```python
from build123d import *

# Parameters (mm, degrees)
SKETCH1_W                    = 400
SKETCH1_H                    = 150
BASE_FLANGE1_DEPTH           = 3
EDGE_FLANGE1_STRIP_W         = 13.4732
EDGE_FLANGE1_STRIP_H         = 3
EDGE_FLANGE1_STRIP_CUT_DEPTH = 400
EDGE_FLANGE1_DEPTH           = 400
EDGE_FLANGE2_STRIP_W         = 13.4732
EDGE_FLANGE2_STRIP_H         = 3
EDGE_FLANGE2_STRIP_CUT_DEPTH = 400
EDGE_FLANGE2_DEPTH           = 400


# Sheet-metal steps are written as plain solids
with BuildPart() as part:
    # Sketch1 → Base-Flange1 (new body)
    with BuildSketch(Plane.XY):
        Rectangle(SKETCH1_W, SKETCH1_H)
    extrude(amount=-BASE_FLANGE1_DEPTH)

    # Edge-Flange1 strip (across the edge) → Edge-Flange1 strip cut (cut)
    with BuildSketch(Plane(origin=(-200, -75, 0), x_dir=(0, 1, 0), z_dir=(1, 0, 0))):
        with Locations((-3, -1.5)):
            Rectangle(EDGE_FLANGE1_STRIP_W, EDGE_FLANGE1_STRIP_H)
    extrude(amount=EDGE_FLANGE1_STRIP_CUT_DEPTH, mode=Mode.SUBTRACT)

    # Edge-Flange1 section (across the edge) → Edge-Flange1 (add)
    with BuildSketch(Plane(origin=(-200, -75, 0), x_dir=(0, 1, 0), z_dir=(1, 0, 0))):
        with BuildLine():
            Line((0, 0.7366), (0, 50.8))
            Line((0, 50.8), (3, 50.8))
            Line((3, 50.8), (3, 0.7366))
            ThreePointArc((3, 0.7366), (3.215745145, 0.215745145), (3.7366, 0))
            Line((3.7366, 0), (3.7366, -3))
            ThreePointArc((3.7366, -3), (1.094424801, -1.905575199), (0, 0.7366))
        make_face()
    extrude(amount=EDGE_FLANGE1_DEPTH)

    # Edge-Flange2 strip (across the edge) → Edge-Flange2 strip cut (cut)
    with BuildSketch(Plane(origin=(200, 75, 0), x_dir=(0, -1, 0), z_dir=(-1, 0, 0))):
        with Locations((-3, -1.5)):
            Rectangle(EDGE_FLANGE2_STRIP_W, EDGE_FLANGE2_STRIP_H)
    extrude(amount=EDGE_FLANGE2_STRIP_CUT_DEPTH, mode=Mode.SUBTRACT)

    # Edge-Flange2 section (across the edge) → Edge-Flange2 (add)
    with BuildSketch(Plane(origin=(200, 75, 0), x_dir=(0, -1, 0), z_dir=(-1, 0, 0))):
        with BuildLine():
            Line((0, 0.7366), (0, 50.8))
            Line((0, 50.8), (3, 50.8))
            Line((3, 50.8), (3, 0.7366))
            ThreePointArc((3, 0.7366), (3.215745145, 0.215745145), (3.7366, 0))
            Line((3.7366, 0), (3.7366, -3))
            ThreePointArc((3.7366, -3), (1.094424801, -1.905575199), (0, 0.7366))
        make_face()
    extrude(amount=EDGE_FLANGE2_DEPTH)


solid = part.part
```
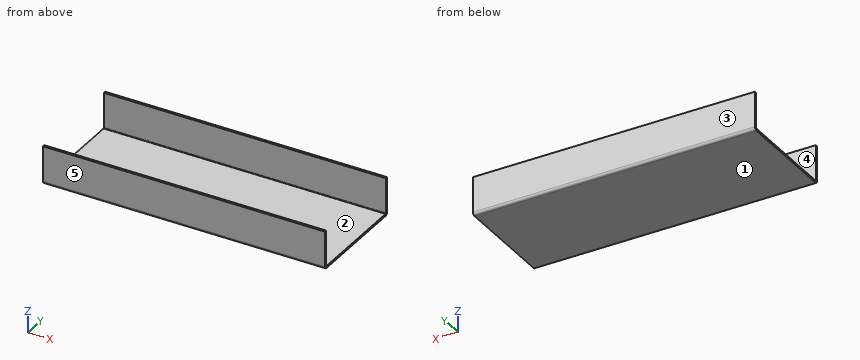
Check sheet for the modelled part. Datum: model origin and axes. Units: mm. Face numbers are marked on the shaded views. A direction names the side the tool comes from. Round coordinates to 2 decimals unless told otherwise and drop trailing zeros. Loops run counter-clockwise (first coordinate to the right, second up) from the corner with the lowest first, then second, coordinate; pieces in that order, holes last. Notation, with made-up numbers: (-0.5, -36.5) -> (29.5, -36.5) arc R24 ccw to (29.5, -20.5) -> close; hole circle Ø2 at (60.5, 17.25). An arc over 180 degrees is marked (long way). Answer in a Markdown table with one row per item.
Q1. Go/stop test with flat-tipped pins: P1, Ø1.5, axis at x = -93.5, y = -12, coming from the +Z side; P2, Ø10, axis at y = 57.5, z = 9, coming from the -X side. Record where each tip stops, or that it passes through.
Data:
| item | result |
|---|---|
| P1 | stops at z = 0 |
| P2 | passes through |
Q2. Sectioned sample at B-B on x = 12.5. Enter the section's corners in (y, z).
Data:
| item | result |
|---|---|
| outline | (-75, 0.74) arc R3.74 ccw to (-71.26, -3) -> (71.26, -3) arc R3.74 ccw to (75, 0.74) -> (75, 50.8) -> (72, 50.8) -> (72, 0.74) arc R0.74 cw to (71.26, 0) -> (-71.26, 0) arc R0.74 cw to (-72, 0.74) -> (-72, 50.8) -> (-75, 50.8) -> close |
Q3. Release check for a two-part mould opening along Y. For the marked faces 3, 4 and 5 record: released by +Y, released by -Y, zero draft, split by the parting line, or undercut.
Data:
| item | result |
|---|---|
| face 3 | released by +Y |
| face 4 | undercut |
| face 5 | released by -Y |
Q4. Sectioned sample at C-C on y = -21. Enter the section's corners in (x, z).
Data:
| item | result |
|---|---|
| outline | (-200, -3) -> (200, -3) -> (200, 0) -> (-200, 0) -> close |
Q5. Thickness scan on L1, parallel to Y at x = 50.5, z = 29.5; L2, parallel to Z at x = -182, y = 52. Record the ranges inside material, lowest first.
Data:
| item | result |
|---|---|
| L1 | y = -75 to -72, 72 to 75 |
| L2 | z = -3 to 0 |
Q6. Sectioned sample at A-A on z = 19. Enter the section's corners in (x, y).
Data:
| item | result |
|---|---|
| outline | (-200, -75) -> (200, -75) -> (200, -72) -> (-200, -72) -> close; (-200, 72) -> (200, 72) -> (200, 75) -> (-200, 75) -> close |
Q7. Set-up check for the marked faces 1 and 2: record each of +Z, -Z, +X, -X, +Y, -Y from which the full face is reachable in a straight line by a thin tool's end or side.
Data:
| item | result |
|---|---|
| face 1 | -Z, +X, -X, +Y, -Y |
| face 2 | +Z, +X, -X |
